from build123d import *

# Parameters (mm, degrees)
SKETCH_1_W          = 60
SKETCH_1_H          = 100
SKETCH_1_R          = 10
EXTRUDE_1_DEPTH     = 10
SKETCH_2_R          = 10
EXTRUDE_2_DEPTH     = 2
FILLET_1_R          = 20
SKETCH_3_W          = 60
SKETCH_3_H          = 50
EXTRUDE_3_DEPTH     = 5
SKETCH_4_R          = 2.25
CUT_EXTRUDE_1_DEPTH = 105.043260233
CUT_EXTRUDE_START   = -10
SKETCH_5_R          = 10
CUT_EXTRUDE_2_DEPTH = 10


with BuildPart() as part:
    # 草图1 → 凸台-拉伸1 (new body)
    with BuildSketch(Plane.XY):
        with Locations((0, 50)):
            Rectangle(SKETCH_1_W, SKETCH_1_H)
        with Locations((0, 80)):
            Circle(SKETCH_1_R, mode=Mode.SUBTRACT)
    extrude(amount=EXTRUDE_1_DEPTH)

    # 草图2 → 凸台-拉伸2 (add)
    with BuildSketch(Plane(origin=(0, 0, 0), x_dir=(-1, 0, 0), z_dir=(0, 0, -1))):
        with Locations((0, 80)):
            Circle(SKETCH_2_R)
    extrude(amount=-EXTRUDE_2_DEPTH)

    # 圆角1
    fillet_1_edges = [part.edges().sort_by_distance(p)[0] for p in [
        (-30, 100, 5),
        (30, 100, 5),
    ]]
    fillet(fillet_1_edges, radius=FILLET_1_R)

    # 草图3 → 凸台-拉伸3 (add)
    with BuildSketch(Plane.XZ):
        with Locations((0, 5)):
            Rectangle(SKETCH_3_W, SKETCH_3_H)
    extrude(amount=-EXTRUDE_3_DEPTH)

    # 草图4 → 切除-拉伸1 (cut, through all)
    with BuildSketch(Plane(origin=(0, 5, 0), x_dir=(1, 0, 0), z_dir=(0, 1, 0))):
        with Locations(Location((-20, 10, 0), (0, 0, 270))):
            Circle(SKETCH_4_R)
        with Locations(Location((20, 10, 0), (0, 0, 270))):
            Circle(SKETCH_4_R)
        with Locations(Location((-20, -20, 0), (0, 0, 270))):
            Circle(SKETCH_4_R)
        with Locations(Location((20, -20, 0), (0, 0, 270))):
            Circle(SKETCH_4_R)
    extrude(amount=-CUT_EXTRUDE_1_DEPTH, mode=Mode.SUBTRACT)

    # 草图5 → 切除-拉伸2 (cut)
    with BuildSketch(Plane.XY.offset(2).offset(CUT_EXTRUDE_START)):
        with Locations((0, 80)):
            Circle(SKETCH_5_R)
    extrude(amount=CUT_EXTRUDE_2_DEPTH, mode=Mode.SUBTRACT)


solid = part.part
Could you check a few things on this model? Use its own coordinates, in mm. A direction names the side the tool comes from. Give positions to 0.01 mm unless a question says otherwise; leave off trailing zeros. Order: outer loops, then holes, each group sorted by start corner. A loop starts at its lowest first (then second) coordinate and runs counter-clockwise, first axis right, second up. Notation, with made-up numbers: (-8.5, -14) - (16.5, -14) arc R17 ccw to (16.5, 8) - close; hole circle Ø3 at (-14.75, 60.25). An arc over 180 degrees is marked (long way). One line per question, with ' | ' between items. Start each with the question number.
Item 1: I want a section at A-A on x = 0. Write out the boundary of the cut face in (y, z), then the cut area to 3 significant figures.
Item 2: I need wall thicknesses on probe 1 along X at (y, z) = (1, -10); probe 2 along X at (y, z) = (80, 7); probe 3 along Y at (x, z) = (-26, -2). Which ranges of each line are inside material? Lowest first, please. Write a range as [from, to].
Item 3: I want a section at C-C on z = 2. Write out the boundary of the cut face in (x, y), then the cut area to 3 significant figures.
Item 4: I'm going to push flat-ended pins straight in: pin 1 Ø18 at (x, y) = (5.5, 64) entering from +Z; pin 2 Ø7 at (x, z) = (-20, -10) entering from +Y; pin 3 Ø3.5 at (x, z) = (20, 20) entering from +Y. Where does each tip first touch, or does it pass through?
Item 5: I want a section at D-D on x = 8. Write out the boundary of the cut face in (y, z).
Item 6: I want a section at B-B on z = 20. Write out the boundary of the cut face in (x, y), then the cut area to 3 significant figures.
Item 7: For faces 4 (the flat face through (0, 53, 10)), 5 (the flat face through (0, 2, -20)), 6 (the flat face through (0, 53, 0)), which set-ups out of +Z, -Z, +X, -X, +Y, -Y let a thin tool reach every point of the face, with its end or its side?
Item 8: Thinking about a two-plate mould opening in Z: for faces 1 (the flat face through (0, 2, 30)), 2 (the flat face through (0, 5, 20)), 3 (the cylindrical face through (-22.196, 2.535, -10.488)), which applies, pulls with the +Z half, pulls with the -Z half, needs draft (parallel to the pull), parting line crosses it, or undercut?
Verdict:
1) outline: (0, -20) - (5, -20) - (5, 0) - (70, 0) - (70, 10) - (5, 10) - (5, 30) - (0, 30) - close; (90, 0) - (100, 0) - (100, 10) - (90, 10) - close | area: 1,000 mm^2
2) probe 1: [-30, -22.25], [-17.75, 17.75], [22.25, 30] | probe 2: [-30, -10], [10, 30] | probe 3: [0, 5]
3) outline: (-30, 0) - (30, 0) - (30, 80) arc R20 ccw to (10, 100) - (-10, 100) arc R20 ccw to (-30, 80) - close; hole circle Ø20 at (0, 80) | area: 5,510 mm^2
4) pin 1: z = 10 | pin 2: y = 5 | pin 3: through
5) outline: (0, -20) - (5, -20) - (5, 0) - (74, 0) - (74, 10) - (5, 10) - (5, 30) - (0, 30) - close; (86, 0) - (100, 0) - (100, 10) - (86, 10) - close
6) outline: (-30, 0) - (-22.25, 0) - (-22.25, 5) - (-30, 5) - close; (-17.75, 0) - (17.75, 0) - (17.75, 5) - (-17.75, 5) - close; (22.25, 0) - (30, 0) - (30, 5) - (22.25, 5) - close | area: 255 mm^2
7) face 4: +Z, +X, -X, +Y | face 5: -Z, +X, -X, +Y, -Y | face 6: -Z, +X, -X, +Y
8) face 1: pulls with the +Z half | face 2: needs draft | face 3: undercut
